The listing builds one solid part. Answer for the finished solid, in the listing's coordinates (mm). Coordinates: 2 decimals unless noted, no trailing zeros. Loops run counter-clockwise (first coordinate to the right, second up) from the corner with the lowest first, then second, coordinate; pieces in that order, holes last. Notation, with made-up numbers: (25.5, -8) - (44.5, -8) arc R20 ccw to (44.5, 23) - close; hole circle Ø5 at (88, 0.5). An arc over 180 degrees is marked (long way). Put each result on its own line as item: value.
```python
from build123d import *

# Parameters (mm, degrees)
SKETCH_1_R               = 1.6
SKETCH_1_R_2             = 2.05
EXTRUDE_1_DEPTH          = 3
HOLE_WIZARD_2_AT_2_COUNT = 2
HOLE_WIZARD_2_AT_2_PITCH = 25
FILLET_1_R               = 7
CUT_EXTRUDE_1_DEPTH      = 10
FILLET_2_R               = 1
CHAMFER_1_SIZE           = 15
FILLET_3_R               = 5
FILLET_4_R               = 3


with BuildPart() as part:
    # 草图1 → 凸台-拉伸1 (new body)
    with BuildSketch(Plane(origin=(0, 0, 0), x_dir=(0, 0, -1), z_dir=(1, 0, 0))):
        with BuildLine():
            Line((-17.839745962, 19), (37.5, 19))
            Line((37.5, 19), (37.5, -19.287265359))
            ThreePointArc((37.5, -19.287265359), (42.444079317, -23.554230469), (41.715171734, -30.044192356))
            ThreePointArc((41.715171734, -30.044192356), (33.776357191, -39.966054476), (24.398111919, -48.540238981))
            ThreePointArc((24.398111919, -48.540238981), (17.866480238, -49.660583483), (13.327617661, -44.831907605))
            ThreePointArc((13.327617661, -44.831907605), (6.185514087, -34.135545268), (-5.993117858, -30))
            Line((-5.993117858, -30), (-13.5, -30))
            Line((-13.5, -30), (-31.5, -12))
            Line((-31.5, -12), (-31.5, 19))
            Line((-31.5, 19), (-26.5, 24))
            Line((-26.5, 24), (-17.839745962, 19))
        make_face()
        with Locations((-12.5, 0)):
            Circle(SKETCH_1_R, mode=Mode.SUBTRACT)
        with Locations((12.5, 0)):
            Circle(SKETCH_1_R, mode=Mode.SUBTRACT)
        with Locations((-26, 16)):
            Circle(SKETCH_1_R_2, mode=Mode.SUBTRACT)
        Polygon((-17.701010127, -6), (1.334192463, -6), (10.57179677, -22), (-1.701010127, -22), align=None, mode=Mode.SUBTRACT)
        Polygon((29.5, -6), (29.5, -22), (17.5, -22), (8.262395693, -6), align=None, mode=Mode.SUBTRACT)
        Polygon((27.5, 6), (-14, 6), (-14, 13), (20.5, 13), align=None, mode=Mode.SUBTRACT)
        with BuildLine():
            Line((-21, 5), (-21, -7))
            ThreePointArc((-21, -7), (-23.75, -9.75), (-26.5, -7))
            Line((-26.5, -7), (-26.5, 5))
            ThreePointArc((-26.5, 5), (-23.75, 7.75), (-21, 5))
        make_face(mode=Mode.SUBTRACT)
        with BuildLine():
            ThreePointArc((18.766630925, -41.32851784), (18.395317666, -44.346319435), (21.413119261, -44.717632693))
            ThreePointArc((21.413119261, -44.717632693), (30.23590735, -36.651282249), (37.704519693, -27.317074793))
            ThreePointArc((37.704519693, -27.317074793), (37.135530181, -24.330228474), (34.148683862, -24.899217985))
            ThreePointArc((34.148683862, -24.899217985), (27.096951821, -33.712412026), (18.766630925, -41.32851784))
        make_face(mode=Mode.SUBTRACT)
    extrude(amount=EXTRUDE_1_DEPTH)

    # 草图3 → 打孔尺寸(%根据十字)槽沉头木螺钉的类型2 (revolve, cut)
    with BuildSketch(Plane(origin=(3, 0, -12.5), x_dir=(0, 0, -1), z_dir=(0, 1, 0))):
        Polygon((0, 0), (0, 3), (1.55, 3), (1.55, 1.75), (3.3, 0), align=None)
    hole_wizard_2 = revolve(axis=Axis((9.35, 0, -12.5), (-1, 0, 0)), mode=Mode.SUBTRACT)

    # 打孔尺寸(%根据十字)槽沉头木螺钉的类型2 at 2: 打孔尺寸(%根据十字)槽沉头木螺钉的类型2 ×2
    with Locations(*[(0, 0, i * HOLE_WIZARD_2_AT_2_PITCH) for i in range(1, HOLE_WIZARD_2_AT_2_COUNT)]):
        add(hole_wizard_2, mode=Mode.SUBTRACT)

    # 圆角1
    fillet_1_edges = [part.edges().sort_by_distance(p)[0] for p in [
        (1.5, -19.287265359, -37.5),
    ]]
    fillet(fillet_1_edges, radius=FILLET_1_R)

    # 草图5 → 切除-拉伸1 (cut)
    with BuildSketch(Plane(origin=(3, 0, 0), x_dir=(0, 0, -1), z_dir=(1, 0, 0))):
        with BuildLine():
            Line((-27.015881022, -16.484118978), (-16.951503299, -26.548496701))
            ThreePointArc((-16.951503299, -26.548496701), (-12.720005473, -20.02392536), (-19.242870048, -15.789797024))
            ThreePointArc((-19.242870048, -15.789797024), (-23.108459656, -16.37111358), (-27.015881022, -16.484118978))
        make_face()
    extrude(amount=-CUT_EXTRUDE_1_DEPTH, mode=Mode.SUBTRACT)

    # 圆角2
    fillet_2_edges = [part.edges().sort_by_distance(p)[0] for p in [
        (1.5, -26.548496701, 16.951503299),
        (1.5, -16.484118978, 27.015881022),
    ]]
    fillet(fillet_2_edges, radius=FILLET_2_R)

    # 倒角1
    chamfer_1_edges = [part.edges().sort_by_distance(p)[0] for p in [
        (1.5, 19, -37.5),
    ]]
    chamfer(chamfer_1_edges, length=CHAMFER_1_SIZE)

    # 圆角3
    fillet_3_edges = [part.edges().sort_by_distance(p)[0] for p in [
        (1.5, 19, -22.5),
        (1.5, 4, -37.5),
        (1.5, 24, 26.5),
        (1.5, 19, 17.839745962),
        (1.5, -30, 13.5),
        (1.5, -12, 31.5),
        (1.5, 19, 31.5),
    ]]
    fillet(fillet_3_edges, radius=FILLET_3_R)

    # 圆角4
    fillet_4_edges = [part.edges().sort_by_distance(p)[0] for p in [
        (1.5, -6, 17.701010127),
        (1.5, -22, 1.701010127),
        (1.5, -22, -10.57179677),
        (1.5, -6, -1.334192463),
        (1.5, -22, -17.5),
        (1.5, -22, -29.5),
        (1.5, -6, -29.5),
        (1.5, -6, -8.262395693),
        (1.5, 13, -20.5),
        (1.5, 13, 14),
        (1.5, 6, 14),
        (1.5, 6, -27.5),
    ]]
    fillet(fillet_4_edges, radius=FILLET_4_R)


solid = part.part
```
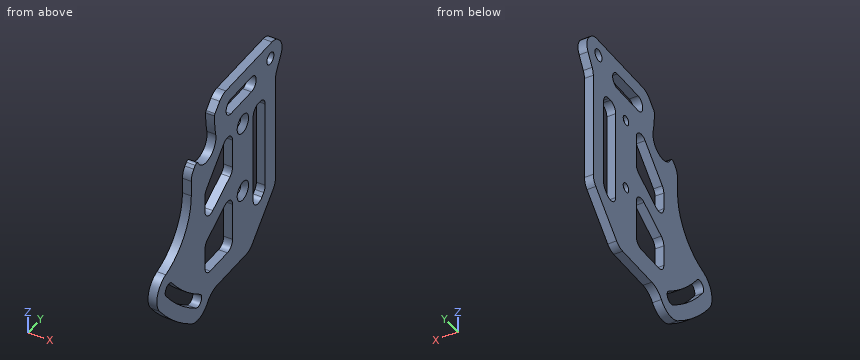
1) The part is cut by section A-A (y = 0). Give the vertices of the cut face in (x, z), and give its area (3 significant figures).
Found:
outline: (0, -37.5) - (3, -37.5) - (3, -15.8) - (1.3, -14.1) - (0, -14.1) - close; (0, -10.9) - (1.3, -10.9) - (3, -9.2) - (3, 9.2) - (1.3, 10.9) - (0, 10.9) - close; (0, 14.1) - (1.3, 14.1) - (3, 15.8) - (3, 21) - (0, 21) - close; (0, 26.5) - (3, 26.5) - (3, 31.5) - (0, 31.5) - close
area: 166 mm^2
2) The part is cut by section D-D (y = -43.5). Give the vertices of the cut face in (x, z).
Found:
outline: (0, -30.26) - (3, -30.26) - (3, -22.93) - (0, -22.93) - close; (0, -17.99) - (3, -17.99) - (3, -12.92) - (0, -12.92) - close
3) Straight lines are drawn through the part: L1, parallel to Z at x = 0.7, y = 0; L2, parallel to Y at x = 0.1, z = 1; L3, parallel to Y at x = 2.25, z = 26. For each, find the intervals that lie inside material, in ascending order. Write a range as [from, to].
Found:
L1: z = [-37.5, -14.1], [-10.9, 10.9], [14.1, 21], [26.5, 31.5]
L2: y = [-30.63, -21.95], [-6, 6], [13, 19]
L3: y = [-16.5, -8.58], [6.58, 13.95], [18.05, 22.74]
4) Each of these flat-tipped pins is pushed along its axis until it touches: pin 1 (1.5 mm diameter, centred on x = 2, z = -10, fed in from +Y); pin 2 (0.9 mm diameter, centred on x = 1, y = -3.5, fed in from -Z); pin 3 (4 mm diameter, centred on y = 0, z = 12.5, fed in from +X). Where does it stop, or does it pass through?
Found:
pin 1: stops at y = 19
pin 2: stops at z = -37.5
pin 3: stops at x = 1.7
5) The part is cut by section C-C (x = 2.3). State how many separate pieces and enclosed holes the cut face has, and give its area (3 significant figures).
Found:
separate pieces: 1
enclosed holes: 8
area: 2,560 mm^2
6) The part is cut by section B-B (y = 16). Give the vertices of the cut face in (x, z).
Found:
outline: (0, -25.5) - (3, -25.5) - (3, 23.95) - (0, 23.95) - close; (0, 28.05) - (3, 28.05) - (3, 31.5) - (0, 31.5) - close
